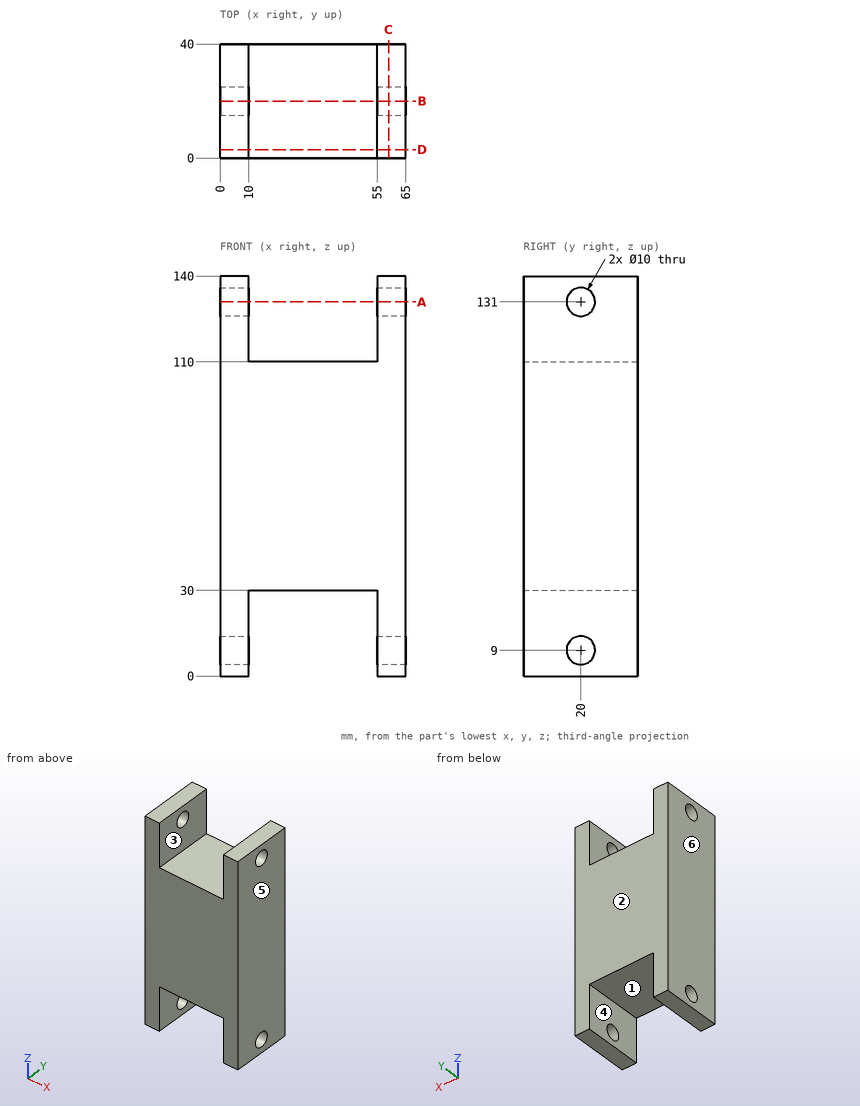
The drawing under review shows one solid part. Ordinate dimensions are in mm from its lowest x, y, z. A direction names the side the tool comes from. Coordinates: 2 decimals unless noted, no trailing zeros. Loops run counter-clockwise (first coordinate to the right, second up) from the corner with the lowest first, then second, coordinate; pieces in that order, holes last. Notation, with made-up numbers: (-35.5, -27) - (-16.5, -27) arc R33 ccw to (-16.5, 6) - close; hole circle Ø8 at (37.25, -32.75). An arc over 180 degrees is marked (long way). Use CSV: the item, a comma, the result in double quotes. Start each with the question number.
1. To check wall thickness, follow probe 1 along X at (y, z) = (3.5, 11); probe 2 along Y at (x, z) = (4, 131); probe 3 along Z at (x, y) = (31, 11). State the ranges of each line that lie inside material, in increasing order.
2. Mouldability with a two-part tool opening along X and no side actions: class the marked faces 4, 5 and 6 as released by +X, released by -X, zero draft, split by the parting line, or undercut.
3. Add section D-D on y = 3. Give the boundary of the cut face in (x, z), plus the area to 3 significant figures.
4. Add section A-A on z = 131. Give the boundary of the cut face in (x, y), plus the area to 3 significant figures.
5. For the marked faces 1, 2 and 3, list the 3-axis set-ups (+Z, -Z, +X, -X, +Y, -Y) from which the entire face can be reached by the end or side of a thin tool; tool diameter is ignored.
6. Add section B-B on y = 20. Give the boundary of the cut face in (x, z), plus the area to 3 significant figures.
7. Clearance check with flat-ended pins moving along their axes: pin 1 (12 mm diameter, centred on x = 27.5, y = 14, fed in from -Z); pin 2 (9 mm diameter, centred on y = 20, z = 9, fed in from +X); pin 3 (6 mm diameter, centred on x = 18, y = 17.5, fed in from +Z). State where each tip first meets the part, or that it passes through.
8. Add section C-C on x = 59. Give the boundary of the cut face in (y, z).
Resolved:
1,probe 1,"0 to 10, 55 to 65"
1,probe 2,"0 to 15, 25 to 40"
1,probe 3,"30 to 110"
2,face 4,"undercut"
2,face 5,"released by +X"
2,face 6,"released by -X"
3,outline,"(0, 0) - (10, 0) - (10, 30) - (55, 30) - (55, 0) - (65, 0) - (65, 140) - (55, 140) - (55, 110) - (10, 110) - (10, 140) - (0, 140) - close"
3,area,"6,400 mm2"
4,outline,"(0, 0) - (10, 0) - (10, 15) - (0, 15) - close; (0, 25) - (10, 25) - (10, 40) - (0, 40) - close; (55, 0) - (65, 0) - (65, 15) - (55, 15) - close; (55, 25) - (65, 25) - (65, 40) - (55, 40) - close"
4,area,"600 mm2"
5,face 1,"-Z, +Y, -Y"
5,face 2,"+Z, -Z, +X, -X, +Y"
5,face 3,"+Z, +Y, -Y"
6,outline,"(0, 0) - (10, 0) - (10, 4) - (0, 4) - close; (0, 14) - (10, 14) - (10, 30) - (55, 30) - (55, 14) - (65, 14) - (65, 126) - (55, 126) - (55, 110) - (10, 110) - (10, 126) - (0, 126) - close; (0, 136) - (10, 136) - (10, 140) - (0, 140) - close; (55, 0) - (65, 0) - (65, 4) - (55, 4) - close; (55, 136) - (65, 136) - (65, 140) - (55, 140) - close"
6,area,"6,000 mm2"
7,pin 1,"z = 30"
7,pin 2,"through"
7,pin 3,"z = 110"
8,outline,"(0, 0) - (40, 0) - (40, 140) - (0, 140) - close; hole circle Ø10 at (20, 9); hole circle Ø10 at (20, 131)"
